Here's how the part is built. I have some questions about the finished solid (model axes, mm). Give positions to 0.01 mm unless a question says otherwise; leave off trailing zeros. Loops run counter-clockwise (first coordinate to the right, second up) from the corner with the lowest first, then second, coordinate; pieces in that order, holes last.
Q1. I need wall thicknesses on probe 1 along Y at (x, z) = (0.3, -14); probe 2 along Y at (x, z) = (0.3, -12.5); probe 3 along Z at (x, y) = (0.8, -2.5). Which ranges of each line are inside material? Lowest first, please.
Q2. Suppose I cut it at A-A (x = 0.5). Count the separate pieces of the cut face and the enclosed holes in it, and give its area (3 significant figures).
Q3. Suppose I cut it at B-B (y = -7.25). List the corners of the cut face in (x, z) for me.
Q4. Suppose I cut it at C-C (z = 8). List the corners of the cut face in (x, y) for me, and give its area (3 significant figures).
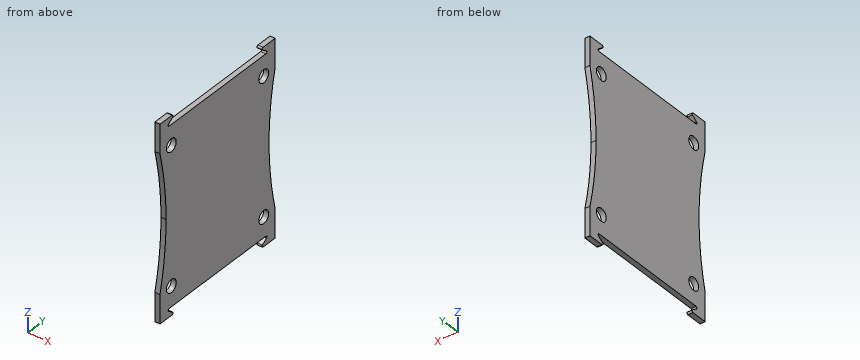
```python
from build123d import *

# Parameters (mm, degrees)
F1_DEPTH = 1
F2_R     = 1.25
F3_DEPTH = 1


with BuildPart() as f1:
    # F0 (on Right) → F1 (new body)
    with BuildSketch(Plane.YZ):
        with BuildLine():
            Line((12.275582, 17.35), (-0.044173, 17.35))
            Line((-0.044173, 17.35), (-12.363928, 17.35))
            ThreePointArc((-12.363928, 17.35), (-12.602005, 17.523717), (-12.509218, 17.803447))
            Line((-12.509218, 17.803447), (-11.468659, 18.546553))
            ThreePointArc((-11.468659, 18.546553), (-11.375872, 18.826283), (-11.613949, 19))
            Line((-11.613949, 19), (-14.694173, 19))
            Line((-14.694173, 19), (-14.694173, 13.4))
            ThreePointArc((-14.694173, 13.4), (-13.532961, 6.744674), (-13.144173, 0))
            ThreePointArc((-13.144173, 0), (-13.532961, -6.744674), (-14.694173, -13.4))
            Line((-14.694173, -13.4), (-14.694173, -19))
            Line((-14.694173, -19), (-11.613949, -19))
            ThreePointArc((-11.613949, -19), (-11.375872, -18.826283), (-11.468659, -18.546553))
            Line((-11.468659, -18.546553), (-12.509218, -17.803447))
            ThreePointArc((-12.509218, -17.803447), (-12.602005, -17.523717), (-12.363928, -17.35))
            Line((-12.363928, -17.35), (-0.044173, -17.35))
            Line((-0.044173, -17.35), (12.275582, -17.35))
            ThreePointArc((12.275582, -17.35), (12.51366, -17.523717), (12.420872, -17.803447))
            Line((12.420872, -17.803447), (11.380313, -18.546553))
            ThreePointArc((11.380313, -18.546553), (11.287526, -18.826283), (11.525603, -19))
            Line((11.525603, -19), (14.605827, -19))
            Line((14.605827, -19), (14.605827, -13.4))
            ThreePointArc((14.605827, -13.4), (13.444615, -6.744674), (13.055827, 0))
            ThreePointArc((13.055827, 0), (13.444615, 6.744674), (14.605827, 13.4))
            Line((14.605827, 13.4), (14.605827, 19))
            Line((14.605827, 19), (11.525603, 19))
            ThreePointArc((11.525603, 19), (11.287526, 18.826283), (11.380313, 18.546553))
            Line((11.380313, 18.546553), (12.420872, 17.803447))
            ThreePointArc((12.420872, 17.803447), (12.51366, 17.523717), (12.275582, 17.35))
        make_face()
    extrude(amount=F1_DEPTH)

    # F2 (on face) → F3 (cut, through all)
    with BuildSketch(Plane.YZ):
        with Locations((11.705827, 13.4)):
            Circle(F2_R)
        with Locations((-11.794173, 13.4)):
            Circle(F2_R)
        with Locations((-11.794173, -13.4)):
            Circle(F2_R)
        with Locations((11.705827, -13.4)):
            Circle(F2_R)
    extrude(amount=F3_DEPTH, mode=Mode.SUBTRACT)


solid = f1.part
```
Solutions:
1. probe 1: y = -14.69 to -12.89, -10.7 to 10.61, 12.8 to 14.61
1. probe 2: y = -14.49 to -12.66, -10.93 to 10.84, 12.57 to 14.4
1. probe 3: z = -17.35 to 17.35
2. separate pieces: 1
2. enclosed holes: 4
2. area: 959 mm2
3. outline: (0, -17.35) - (1, -17.35) - (1, 17.35) - (0, 17.35) - close
4. outline: (0, -13.69) - (1, -13.69) - (1, 13.6) - (0, 13.6) - close
4. area: 27.3 mm2
